from build123d import *

# Parameters (mm, degrees)
SKETCH1_W           = 115
SKETCH1_H           = 60
SKETCH1_R           = 2.1
BOSS_EXTRUDE1_DEPTH = 5
SKETCH2_R           = 4.575
CUT_EXTRUDE1_DEPTH  = 3
SKETCH3_R           = 3.25
CUT_EXTRUDE2_DEPTH  = 0.2
SKETCH4_R           = 1.65
CUT_EXTRUDE3_DEPTH  = 6
CUT_EXTRUDE4_DEPTH  = 6
BOSS_EXTRUDE2_DEPTH = 5
SKETCH8_R           = 1.65
CUT_EXTRUDE5_DEPTH  = 6
FILLET1_R           = 5
SKETCH9_R           = 6
SKETCH9_R_2         = 2.1
BOSS_EXTRUDE3_DEPTH = 2.275
SKETCH10_R          = 2.9
SKETCH10_R_2        = 2.1
BOSS_EXTRUDE4_DEPTH = 0.2
SKETCH11_R          = 3
CUT_EXTRUDE6_DEPTH  = 1


with BuildPart() as part:
    # Sketch1 → Boss-Extrude1 (new body)
    with BuildSketch(Plane(origin=(0, 0, 0), x_dir=(1, 0, 0), z_dir=(0, 1, 0))):
        with Locations((-12.5, 0)):
            Rectangle(SKETCH1_W, SKETCH1_H)
        with Locations((-22, 14)):
            Circle(SKETCH1_R, mode=Mode.SUBTRACT)
        with Locations((0, 18)):
            Circle(SKETCH1_R, mode=Mode.SUBTRACT)
        with Locations((0, -18)):
            Circle(SKETCH1_R, mode=Mode.SUBTRACT)
        with Locations((-22, -14)):
            Circle(SKETCH1_R, mode=Mode.SUBTRACT)
        with Locations((15, -18)):
            Circle(SKETCH1_R, mode=Mode.SUBTRACT)
    extrude(amount=BOSS_EXTRUDE1_DEPTH)

    # Sketch2 → Cut-Extrude1 (cut)
    with BuildSketch(Plane(origin=(0, 5, 0), x_dir=(1, 0, 0), z_dir=(0, 1, 0))):
        Circle(SKETCH2_R)
    extrude(amount=-CUT_EXTRUDE1_DEPTH, mode=Mode.SUBTRACT)

    # Sketch3 → Cut-Extrude2 (cut)
    with BuildSketch(Plane(origin=(0, 2, 0), x_dir=(1, 0, 0), z_dir=(0, 1, 0))):
        Circle(SKETCH3_R)
    extrude(amount=-CUT_EXTRUDE2_DEPTH, mode=Mode.SUBTRACT)

    # Sketch4 → Cut-Extrude3 (cut, through all)
    with BuildSketch(Plane(origin=(0, 5, 0), x_dir=(1, 0, 0), z_dir=(0, 1, 0))):
        with Locations((-34.5, -8)):
            Circle(SKETCH4_R)
        with Locations((-34.5, 8)):
            Circle(SKETCH4_R)
    extrude(amount=-CUT_EXTRUDE3_DEPTH, mode=Mode.SUBTRACT)

    # Sketch6 → Cut-Extrude4 (cut, through all)
    with BuildSketch(Plane(origin=(0, 5, 0), x_dir=(1, 0, 0), z_dir=(0, 1, 0))):
        with BuildLine():
            Line((-22, 18.221576202), (-34.5, 18.221576202))
            ThreePointArc((-34.5, 18.221576202), (-38.035533906, 16.757110108), (-39.5, 13.221576202))
            Line((-39.5, 13.221576202), (-39.5, -13.221576202))
            ThreePointArc((-39.5, -13.221576202), (-38.035533906, -16.757110108), (-34.5, -18.221576202))
            Line((-34.5, -18.221576202), (-22, -18.221576202))
            Line((-22, -18.221576202), (-8.297519941, -18.221576202))
            Line((-8.297519941, -18.221576202), (14.635521586, -36.006383916))
            Line((14.635521586, -36.006383916), (-22, -30))
            Line((-22, -30), (-70, -30))
            Line((-70, -30), (-70, 30))
            Line((-70, 30), (-22, 30))
            Line((-22, 30), (16.094767965, 37.138044373))
            Line((16.094767965, 37.138044373), (-8.297519941, 18.221576202))
            Line((-8.297519941, 18.221576202), (-22, 18.221576202))
        make_face()
    extrude(amount=-CUT_EXTRUDE4_DEPTH, mode=Mode.SUBTRACT)

    # Sketch7 → Boss-Extrude2 (add)
    with BuildSketch(Plane(origin=(0, 5, 0), x_dir=(1, 0, 0), z_dir=(0, 1, 0))):
        Polygon((27.342211368, 39), (15.73694821, 30), (45, 30), (45, 39), align=None)
        Polygon((45, -30), (15.73694821, -30), (27.342211368, -39), (45, -39), align=None)
    extrude(amount=-BOSS_EXTRUDE2_DEPTH)

    # Sketch8 → Cut-Extrude5 (cut, through all)
    with BuildSketch(Plane(origin=(0, 5, 0), x_dir=(1, 0, 0), z_dir=(0, 1, 0))):
        with Locations((35, 32)):
            Circle(SKETCH8_R)
        with Locations((35, -32)):
            Circle(SKETCH8_R)
    extrude(amount=-CUT_EXTRUDE5_DEPTH, mode=Mode.SUBTRACT)

    # Fillet1
    fillet1_edges = [part.edges().sort_by_distance(p)[0] for p in [
        (45, 2.5, -39),
        (27.342211368, 2.5, -39),
        (27.342211368, 2.5, 39),
        (45, 2.5, 39),
        (-8.297519941, 2.5, 18.221576202),
        (-8.297519941, 2.5, -18.221576202),
    ]]
    fillet(fillet1_edges, radius=FILLET1_R)

    # Sketch9 → Boss-Extrude3 (add)
    with BuildSketch(Plane(origin=(0, 5, 0), x_dir=(1, 0, 0), z_dir=(0, 1, 0))):
        with Locations((15, -18)):
            Circle(SKETCH9_R)
        with Locations((15, -18)):
            Circle(SKETCH9_R_2, mode=Mode.SUBTRACT)
    extrude(amount=BOSS_EXTRUDE3_DEPTH)

    # Sketch10 → Boss-Extrude4 (add)
    with BuildSketch(Plane(origin=(0, 7.275, 0), x_dir=(1, 0, 0), z_dir=(0, 1, 0))):
        with Locations((15, -18)):
            Circle(SKETCH10_R)
        with Locations((15, -18)):
            Circle(SKETCH10_R_2, mode=Mode.SUBTRACT)
    extrude(amount=BOSS_EXTRUDE4_DEPTH)

    # Sketch11 → Cut-Extrude6 (cut)
    with BuildSketch(Plane(origin=(0, 5, 0), x_dir=(1, 0, 0), z_dir=(0, 1, 0))):
        with Locations((-34.5, 8)):
            Circle(SKETCH11_R)
        with Locations((-34.5, -8)):
            Circle(SKETCH11_R)
        with Locations((35, -32)):
            Circle(SKETCH11_R)
        with Locations((35, 32)):
            Circle(SKETCH11_R)
    extrude(amount=-CUT_EXTRUDE6_DEPTH, mode=Mode.SUBTRACT)


solid = part.part
Geometry check sheet. Reference: the model listing, model coordinates, mm. A direction names the side the tool comes from. Give positions to 0.01 mm unless a question says otherwise; leave off trailing zeros. Write each loop counter-clockwise with the first axis right and the second up, starting at its lowest first coordinate (ties: lowest second). Pieces come first, ordered by that corner, then holes. Notation, with made-up numbers: M -7,10.25 L 9,10.25 A22 cw 9,45.25 Z; hole C 61,37 d2. An arc over 180 degrees is marked long. Answer as CSV lines item,"result". Start each with the question number.
Q1. Section check C-C, the plane y = 6.25. Record the cut outline in (x, z), then the cut area to 3 significant figures.
Q2. Release check for a two-part mould opening along X. For faces 1 (the face through (-39.5, 3, 0)), 2 (the face through (44, 2, 37)), 3 (the face through (12, 5, -1)), 4 (the face through (36.3, 4, -30.7)) record: pulls with the +X half, pulls with the -X half, needs draft (parallel to the pull), parting line crosses it, or undercut.
Q3. Section check A-A, the plane x = -22. Record the cut outline in (y, z), then the cut area to 3 significant figures.
Q4. Section check B-B, the plane x = 0. Record the cut outline in (y, z) (3 decimals), then the cut area to 3 significant figures.
Q5. Tool access check on faces 5 (the face through (-0.273, 2.465, 15.918)), 6 (the face through (34, 3, 39)), 7 (the face through (-33, 4, 9)), 8 (the face through (11, 2, 30)), 9 (the face through (11, 2, -30)). Record the directions out of +Z, -Z, +X, -X, +Y, -Y that give a thin tool (end or side, any length) a straight path to the whole face; none if there is none.
Q6. Section check D-D, the plane z = 23. Record the cut outline in (x, y) (3 decimals), then the cut area to 3 significant figures.
Q7. Material ranges on L1, parallel to Z at x = -22, y = 3.75; L2, parallel to Z at x = -34.5, y = 4.6; L3, parallel to Y at x = 23, z = 16, recorded low to high.
Q8. Go/stop test with flat-tipped pins: pin 1 (5 mm diameter, centred on x = -1.5, z = -0.5, fed in from +Y); pin 2 (6.5 mm diameter, centred on x = 35, z = 31, fed in from +Y); pin 3 (2.5 mm diameter, centred on x = -23.5, y = 1.5, fed in from -Z); pin 4 (4 mm diameter, centred on x = -34.5, z = -8, fed in from -Y). Record where each tip stops, or that it passes through.
Geometry says:
1,outline,"C 15,18 d12; hole C 15,18 d4.2"
1,area,"99.2 mm^2"
2,face 1,"pulls with the -X half"
2,face 2,"pulls with the +X half"
2,face 3,"needs draft"
2,face 4,"undercut"
3,outline,"M 0,-18.22 L 5,-18.22 L 5,-16.1 L 0,-16.1 Z; M 0,-11.9 L 5,-11.9 L 5,11.9 L 0,11.9 Z; M 0,16.1 L 5,16.1 L 5,18.22 L 0,18.22 Z"
3,area,"140 mm^2"
4,outline,"M 0,-24.656 L 5,-24.656 L 5,-20.1 L 0,-20.1 Z; M 0,-15.9 L 5,-15.9 L 5,-4.575 L 2,-4.575 L 2,-3.25 L 1.8,-3.25 L 1.8,3.25 L 2,3.25 L 2,4.575 L 5,4.575 L 5,15.9 L 0,15.9 Z; M 0,20.1 L 5,20.1 L 5,24.656 L 0,24.656 Z"
4,area,"176 mm^2"
5,face 5,"+Y, -Y"
5,face 6,"+Z, +X, -X, +Y, -Y"
5,face 7,"+Y"
5,face 8,"+Z, -X, +Y, -Y"
5,face 9,"-Z, -X, +Y, -Y"
6,outline,"M -2.136,0 L 45,0 L 45,5 L 18.317,5 L 18.317,7.275 L 11.683,7.275 L 11.683,5 L -2.136,5 Z"
6,area,"251 mm^2"
7,L1,"-18.22 to -16.1, -11.9 to 11.9, 16.1 to 18.22"
7,L2,"-18.22 to -11, -5 to 5, 11 to 18.22"
7,L3,"0 to 5"
8,pin 1,"y = 2"
8,pin 2,"y = 5"
8,pin 3,"z = -18.22"
8,pin 4,"y = 0"
